Verification items for the finished model (mm, model axes). Round coordinates to 2 decimals unless told otherwise and drop trailing zeros. Write each loop counter-clockwise with the first axis right and the second up, starting at its lowest first coordinate (ties: lowest second). Pieces come first, ordered by that corner, then holes. Notation, with made-up numbers: (63.5, 53) - (105.5, 53) arc R11 ccw to (105.5, 61) - close; hole circle Ø5 at (-2, 12.25). An arc over 180 degrees is marked (long way). Answer as a JSON object with one key per item and string values. Group by question number.
1) Section check C-C (y = 20). Enter the section's corners in (x, z), then the cut area to 3 significant figures.
2) Section check A-A (x = 7). Enter the section's corners in (y, z).
3) Section check B-B (z = -200). Enter the section's corners in (x, y), then the cut area to 3 significant figures.
4) Section check D-D (z = -96). Enter the section's corners in (x, y).
5) Thickness scan on line 1 (Y direction, x = 7, z = -110); line 2 (Y direction, x = 2.5, z = -20); line 3 (Y direction, x = 6, z = -184.5). Record the ranges inside material, lowest first.
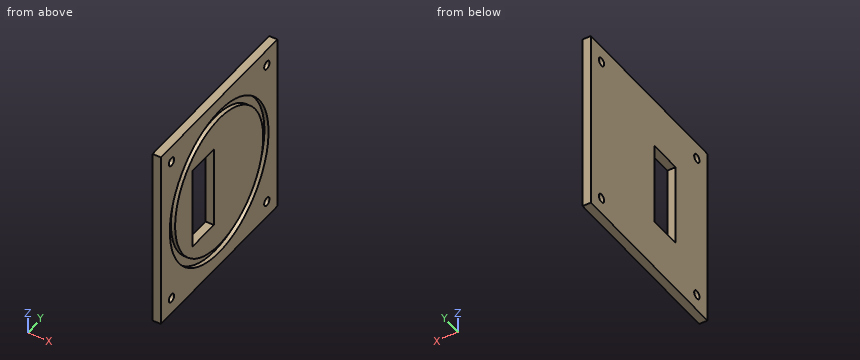
```python
from build123d import *

# Parameters (mm, degrees)
SKETCH1_W           = 220
SKETCH1_H           = 220
SKETCH1_W_2         = 100
SKETCH1_H_2         = 40
BOSS_EXTRUDE1_DEPTH = 10
SKETCH2_R           = 93.17284
SKETCH2_R_2         = 83.17284
CUT_EXTRUDE1_DEPTH  = 5
SKETCH3_R           = 5
CUT_EXTRUDE2_DEPTH  = 11


with BuildPart() as part:
    # Sketch1 → Boss-Extrude1 (new body)
    with BuildSketch(Plane(origin=(0, 0, 0), x_dir=(0, 0, -1), z_dir=(1, 0, 0))):
        with Locations((110, 110)):
            Rectangle(SKETCH1_W, SKETCH1_H)
        with Locations((110, 80)):
            Rectangle(SKETCH1_W_2, SKETCH1_H_2, mode=Mode.SUBTRACT)
    extrude(amount=BOSS_EXTRUDE1_DEPTH)

    # Sketch2 → Cut-Extrude1 (cut)
    with BuildSketch(Plane(origin=(10, 0, 0), x_dir=(0, 0, -1), z_dir=(1, 0, 0))):
        with Locations((110, 110)):
            Circle(SKETCH2_R)
        with Locations((110, 110)):
            Circle(SKETCH2_R_2, mode=Mode.SUBTRACT)
    extrude(amount=-CUT_EXTRUDE1_DEPTH, mode=Mode.SUBTRACT)

    # Sketch3 → Cut-Extrude2 (cut, through all)
    with BuildSketch(Plane(origin=(10, 0, 0), x_dir=(0, 0, -1), z_dir=(1, 0, 0))):
        with Locations((20, 200)):
            Circle(SKETCH3_R)
        with Locations((200, 200)):
            Circle(SKETCH3_R)
        with Locations((200, 20)):
            Circle(SKETCH3_R)
        with Locations((20, 20)):
            Circle(SKETCH3_R)
    extrude(amount=-CUT_EXTRUDE2_DEPTH, mode=Mode.SUBTRACT)


solid = part.part
```
Returned:
{
 "1": {"outline": "(0, -220) - (10, -220) - (10, -205) - (0, -205) - close; (0, -195) - (10, -195) - (10, -134.11) - (5, -134.11) - (5, -85.89) - (10, -85.89) - (10, -25) - (0, -25) - close; (0, -15) - (10, -15) - (10, 0) - (0, 0) - close", "area": "1,760 mm2"},
 "2": {"outline": "(0, -220) - (220, -220) - (220, 0) - (0, 0) - close; circle Ø166.35 at (110, -110); hole circle Ø10 at (20, -200); hole circle Ø10 at (20, -20); hole circle Ø186.35 at (110, -110); hole (60, -160) - (100, -160) - (100, -60) - (60, -60) - close; hole circle Ø10 at (200, -200); hole circle Ø10 at (200, -20)"},
 "3": {"outline": "(0, 0) - (10, 0) - (10, 15) - (0, 15) - close; (0, 25) - (10, 25) - (10, 85.89) - (5, 85.89) - (5, 134.11) - (10, 134.11) - (10, 195) - (0, 195) - close; (0, 205) - (10, 205) - (10, 220) - (0, 220) - close", "area": "1,760 mm2"},
 "4": {"outline": "(0, 0) - (10, 0) - (10, 17.88) - (5, 17.88) - (5, 28.01) - (10, 28.01) - (10, 60) - (0, 60) - close; (0, 100) - (10, 100) - (10, 191.99) - (5, 191.99) - (5, 202.12) - (10, 202.12) - (10, 220) - (0, 220) - close"},
 "5": {"line 1": "0 to 16.83, 26.83 to 60, 100 to 193.17, 203.17 to 220", "line 2": "0 to 15, 25 to 195, 205 to 220", "line 3": "0 to 54.05, 73.02 to 146.98, 165.95 to 220"}
}
